from build123d import *

# Parameters (mm, degrees)
SKETCH3_R               = 15.55
SKETCH3_R_2             = 8.15
BOSS_EXTRUDE4_DEPTH     = 6.5
SKETCH2_R               = 15.55
SKETCH2_R_2             = 8.15
BOSS_EXTRUDE5_DEPTH     = 6.5
CUT_EXTRUDE1_DEPTH      = 35.8
SKETCH5_R               = 1.6
CUT_EXTRUDE2_DEPTH      = 43.014818814
BOSS_EXTRUDE6_DEPTH     = 6.5
SKETCH9_W               = 6.5
SKETCH9_H               = 21.954006421
BOSS_EXTRUDE7_DEPTH     = 4
BOSS_EXTRUDE8_DEPTH     = 6.5
FILLET1_R               = 2
FILLET5_R               = 2
CUT_EXTRUDE3_DEPTH      = 47.905543459
BOSS_EXTRUDE10_START    = -6.5
SKETCH13_W              = 19.5
SKETCH13_H              = 7.8
BOSS_EXTRUDE10_DEPTH    = 35.8
FILLET3_R               = 2
SKETCH14_W              = 19.5
SKETCH14_H              = 5
BOSS_EXTRUDE11_DEPTH    = 5
CUT_EXTRUDE4_DEPTH      = 62.410850086
SKETCH20_W              = 19.5
SKETCH20_H              = 5
BOSS_EXTRUDE13_DEPTH    = 4.5
SKETCH21_R              = 1.6
CUT_EXTRUDE7_DEPTH      = 62.410850086
FILLET6_R               = 1
SKETCH22_R              = 2.35
CUT_EXTRUDE8_DEPTH      = 10
SKETCH23_R              = 1.6
CUT_EXTRUDE9_DEPTH      = 54.54433838
CUT_EXTRUDE9_DEPTH_BACK = 54.54433838


with BuildPart() as part:
    # Sketch3 → Boss-Extrude4 (new body)
    with BuildSketch(Plane(origin=(0, 0, 0), x_dir=(0, 0, -1), z_dir=(1, 0, 0))):
        with Locations(Location((0, 0, 0), (0, 0, 180))):
            Circle(SKETCH3_R)
        with Locations(Location((0, 0, 0), (0, 0, 180))):
            Circle(SKETCH3_R_2, mode=Mode.SUBTRACT)
    extrude(amount=BOSS_EXTRUDE4_DEPTH)


with BuildPart() as body_2:
    # Sketch2 → Boss-Extrude5 (new body)
    with BuildSketch(Plane(origin=(35.8, 0, 0), x_dir=(0, 0, -1), z_dir=(1, 0, 0))):
        Circle(SKETCH2_R)
        Circle(SKETCH2_R_2, mode=Mode.SUBTRACT)
    extrude(amount=-BOSS_EXTRUDE5_DEPTH)


with BuildPart() as cut_extrude1_tool:
    # Sketch4 → Cut-Extrude1 (new body)
    with BuildSketch(Plane(origin=(0, 0, 0), x_dir=(0, 0, -1), z_dir=(1, 0, 0))):
        with BuildLine():
            Line((0, 15.55), (0, -15.55))
            ThreePointArc((0, -15.55), (15.55, 0), (0, 15.55))
        make_face()
    extrude(amount=CUT_EXTRUDE1_DEPTH)


with BuildPart() as part_1:
    add(part.part)

    # Cut-Extrude1: cut by cut_extrude1_tool
    add(cut_extrude1_tool.part, mode=Mode.SUBTRACT)


with BuildPart() as body_2_1:
    add(body_2.part)

    # Cut-Extrude1: cut by cut_extrude1_tool
    add(cut_extrude1_tool.part, mode=Mode.SUBTRACT)


with BuildPart() as cut_extrude2_tool:
    # Sketch5 → Cut-Extrude2 (new, through all)
    with BuildSketch(Plane(origin=(0, 0, 0), x_dir=(-1, 0, 0), z_dir=(0, 0, -1))):
        with Locations((-32.55, 11.85)):
            Circle(SKETCH5_R)
        with Locations((-3.25, 11.85)):
            Circle(SKETCH5_R)
    extrude(amount=-CUT_EXTRUDE2_DEPTH)


with BuildPart() as part_2:
    add(part_1.part)

    # Cut-Extrude2: cut by cut_extrude2_tool
    add(cut_extrude2_tool.part, mode=Mode.SUBTRACT)

    # Sketch11 → Boss-Extrude8 (add)
    with BuildSketch(Plane.ZY):
        with BuildLine():
            ThreePointArc((15.5, -1.245993579), (10.545788255, -11.427547859), (0, -15.55))
            Line((0, -15.55), (0, -23.2))
            Line((0, -23.2), (19.5, -23.2))
            Line((19.5, -23.2), (19.5, -1.245993579))
            Line((19.5, -1.245993579), (15.5, -1.245993579))
        make_face()
    extrude(amount=-BOSS_EXTRUDE8_DEPTH)

    # Fillet5
    fillet5_edges = [part_2.edges().sort_by_distance(p)[0] for p in [
        (3.25, -1.245993579, 15.5),
    ]]
    fillet(fillet5_edges, radius=FILLET5_R)


with BuildPart() as body_2_2:
    add(body_2_1.part)

    # Cut-Extrude2: cut by cut_extrude2_tool
    add(cut_extrude2_tool.part, mode=Mode.SUBTRACT)

    # Sketch8 → Boss-Extrude6 (add)
    with BuildSketch(Plane.ZY.offset(-29.3)):
        with BuildLine():
            ThreePointArc((15.5, -11.330931118), (8.691551143, -17.120074145), (0, -19.2))
            Line((0, -19.2), (0, -23.2))
            Line((0, -23.2), (15.5, -23.2))
            Line((15.5, -23.2), (15.5, -11.330931118))
        make_face()
        with BuildLine():
            ThreePointArc((15.5, -1.245993579), (10.545788255, -11.427547859), (0, -15.55))
            Line((0, -15.55), (0, -19.2))
            ThreePointArc((0, -19.2), (8.691551143, -17.120074145), (15.5, -11.330931118))
            Line((15.5, -11.330931118), (15.5, -1.245993579))
        make_face()
    extrude(amount=-BOSS_EXTRUDE6_DEPTH)

    # Sketch9 → Boss-Extrude7 (add)
    with BuildSketch(Plane(origin=(0, 0, 15.5), x_dir=(-1, 0, 0), z_dir=(0, 0, -1))):
        with Locations((-32.55, -12.22299679)):
            Rectangle(SKETCH9_W, SKETCH9_H)
    extrude(amount=-BOSS_EXTRUDE7_DEPTH)

    # Fillet1
    fillet1_edges = [body_2_2.edges().sort_by_distance(p)[0] for p in [
        (32.55, -1.245993579, 15.5),
    ]]
    fillet(fillet1_edges, radius=FILLET1_R)


with BuildPart() as cut_extrude3_tool:
    # Sketch10 → Cut-Extrude3 (new, through all)
    with BuildSketch(Plane.ZY.offset(-35.8)):
        with BuildLine():
            Line((19.5, -1.245993579), (19.5, -3.212198374))
            ThreePointArc((19.5, -3.212198374), (18.924111949, -1.82188163), (17.533795206, -1.245993579))
            Line((17.533795206, -1.245993579), (19.5, -1.245993579))
        make_face()
    extrude(amount=CUT_EXTRUDE3_DEPTH)


with BuildPart() as part_3:
    add(part_2.part)

    # Cut-Extrude3: cut by cut_extrude3_tool
    add(cut_extrude3_tool.part, mode=Mode.SUBTRACT)



with BuildPart() as body_2_3:
    add(body_2_2.part)

    # Cut-Extrude3: cut by cut_extrude3_tool
    add(cut_extrude3_tool.part, mode=Mode.SUBTRACT)


with BuildPart() as part_4:
    add(part_3.part)

    add(body_2_3.part)  # Boss-Extrude10 merges body 2
    # Sketch13 → Boss-Extrude10 (add)
    with BuildSketch(Plane.ZY.offset(-29.3).offset(BOSS_EXTRUDE10_START)):
        with Locations((9.75, -27.1)):
            Rectangle(SKETCH13_W, SKETCH13_H)
    extrude(amount=BOSS_EXTRUDE10_DEPTH)

    # Fillet3
    fillet3_edges = [part_4.edges().sort_by_distance(p)[0] for p in [
        (6.5, -23.2, 9.75),
        (29.3, -23.2, 9.75),
    ]]
    fillet(fillet3_edges, radius=FILLET3_R)

    # Sketch14 → Boss-Extrude11 (add)
    with BuildSketch(Plane.ZY.offset(-35.8)):
        with Locations((9.75, -28.5)):
            Rectangle(SKETCH14_W, SKETCH14_H)
    extrude(amount=-BOSS_EXTRUDE11_DEPTH)

    # Sketch15 → Cut-Extrude4 (cut, through all)
    with BuildSketch(Plane(origin=(0, -26, 0), x_dir=(1, 0, 0), z_dir=(0, 1, 0))):
        with BuildLine():
            ThreePointArc((39.9, -9.75), (39.43137085, -8.61862915), (38.3, -8.15))
            Line((38.3, -8.15), (38.3, -11.35))
            ThreePointArc((38.3, -11.35), (39.43137085, -10.88137085), (39.9, -9.75))
        make_face()
        with BuildLine():
            Line((38.3, -11.35), (38.3, -8.15))
            ThreePointArc((38.3, -8.15), (36.7, -9.75), (38.3, -11.35))
        make_face()
    extrude(amount=-CUT_EXTRUDE4_DEPTH, mode=Mode.SUBTRACT)

    # Sketch20 → Boss-Extrude13 (add)
    with BuildSketch(Plane.ZY):
        with Locations((9.75, -28.5)):
            Rectangle(SKETCH20_W, SKETCH20_H)
    extrude(amount=BOSS_EXTRUDE13_DEPTH)

    # Sketch21 → Cut-Extrude7 (cut, through all)
    with BuildSketch(Plane(origin=(0, -26, 0), x_dir=(1, 0, 0), z_dir=(0, 1, 0))):
        with Locations(Location((-2.25, -9.75, 0), (0, 0, 270))):
            Circle(SKETCH21_R)
    extrude(amount=-CUT_EXTRUDE7_DEPTH, mode=Mode.SUBTRACT)

    # Fillet6
    fillet6_edges = [part_4.edges().sort_by_distance(p)[0] for p in [
        (0, 11.229228387, 10.756715569),
        (0, -1.82188163, 18.924111949),
        (29.3, -12.206099187, 19.5),
        (17.9, -23.2, 19.5),
        (6.5, -12.206099187, 19.5),
        (28.714213562, -22.614213562, 19.5),
        (7.085786438, -22.614213562, 19.5),
        (40.8, -28.5, 19.5),
        (38.3, -26, 19.5),
        (-2.25, -26, 19.5),
        (-4.5, -28.5, 19.5),
        (35.8, 11.229228387, 10.756715569),
        (29.3, 11.229228387, 10.756715569),
        (29.3, -0.690267327, 16.150294811),
        (35.8, -0.690267327, 16.150294811),
        (35.8, -14.606099187, 19.5),
        (35.8, -1.82188163, 18.924111949),
        (29.3, -1.82188163, 18.924111949),
        (0, -14.606099187, 19.5),
        (18.15, -31, 19.5),
        (6.5, -0.690267327, 16.150294811),
        (6.5, -1.82188163, 18.924111949),
        (6.5, 11.229228387, 10.756715569),
        (0, -0.690267327, 16.150294811),
    ]]
    fillet(fillet6_edges, radius=FILLET6_R)

    # Sketch22 → Cut-Extrude8 (cut)
    with BuildSketch(Plane(origin=(0, 0, 0), x_dir=(-1, 0, 0), z_dir=(0, 0, -1))):
        with Locations((-8.5, -27.1)):
            Circle(SKETCH22_R)
        with Locations((-27.3, -27.1)):
            Circle(SKETCH22_R)
    extrude(amount=-CUT_EXTRUDE8_DEPTH, mode=Mode.SUBTRACT)

    # Sketch23 → Cut-Extrude9 (cut, two sides)
    with BuildSketch(Plane.XY.offset(15.535641906)) as cut_extrude9_sk:
        with Locations((3.25, 0)):
            Circle(SKETCH23_R)
        with Locations((32.55, 0)):
            Circle(SKETCH23_R)
    extrude(amount=CUT_EXTRUDE9_DEPTH, mode=Mode.SUBTRACT)
    extrude(cut_extrude9_sk.sketch, amount=-CUT_EXTRUDE9_DEPTH_BACK, mode=Mode.SUBTRACT)


solid = part_4.part
Could you check a few things on this model? Use its own coordinates, in mm. A direction names the side the tool comes from. Round coordinates to 2 decimals unless told otherwise and drop trailing zeros. Order: outer loops, then holes, each group sorted by start corner. A loop starts at its lowest first (then second) coordinate and runs counter-clockwise, first axis right, second up.
(1) Please list where these lines run through material, in increasing order: line 1 along X through (y, z) = (0, 14); line 2 along X through (y, z) = (-9.5, 17.5); line 3 along Y through (x, z) = (8.5, 6.75).
Response values:
line 1: x = 0 to 1.65, 4.85 to 6.5, 29.3 to 30.95, 34.15 to 35.8
line 2: x = 0 to 6.5, 29.3 to 35.8
line 3: y = -31 to -29.45, -24.75 to -23.2
(2) Imagine slicing it at C-C (x = 3.25). Write out the boundary of the cut face in (y, z), plus the area to 3 significant figures.
Response values:
outline: (-31, 0) - (-8.15, 0) arc R8.15 cw to (-1.6, 7.99) - (-1.6, 18.66) arc R1.97 ccw to (-3.21, 19.5) - (-30, 19.5) arc R1 ccw to (-31, 18.5) - close; (1.6, 7.99) arc R8.15 cw to (8.15, 0) - (10.25, 0) - (10.25, 11.69) arc R15.55 ccw to (1.6, 15.47) - close; (13.45, 0) - (15.55, 0) arc R15.55 ccw to (13.45, 7.8) - close
area: 627 mm2
(3) Imagine slicing it at D-D (z = 2.75). Count the separate pieces of the cut face and the enclosed holes in it, plus the area to 3 significant figures.
Response values:
separate pieces: 3
enclosed holes: 4
area: 578 mm2
(4) I'm going to push flat-ended pins straight in: pin 1 (9 mm diameter, centred on y = -10, z = 6.5, fed in from -X); pin 2 (8 mm diameter, centred on y = -11, z = 10, fed in from +X); pin 3 (1 mm diameter, centred on x = 36, y = -3, fed in from -Z); pin 4 (8 mm diameter, centred on x = 12, y = -14.5, fed in from -Z). Where does each tip first touch, or does it pass through?
Response values:
pin 1: stops at x = 0
pin 2: stops at x = 35.8
pin 3: stops at z = 7.38
pin 4: passes through
(5) Which directions (+Z, -Z, +X, -X, +Y, -Y) give clear straight access to the entire face, cutting with the end or side of a thin tool? Please do faces 1 (the flat face through (6.5, -7, 9)), 2 (the cylindrical face through (10.365, -28.53, 4.93)), 3 (the flat face through (0, -10, 9)).
Response values:
face 1: +Z, -Z, +Y
face 2: -Z
face 3: +Z, -Z, -X, +Y
(6) Imagine slicing it at A-A (x = -2.25). Write out the boundary of the cut face in (y, z).
Response values:
outline: (-31, 0) - (-26, 0) - (-26, 8.15) - (-31, 8.15) - close; (-31, 11.35) - (-26, 11.35) - (-26, 18.5) arc R1 ccw to (-27, 19.5) - (-30, 19.5) arc R1 ccw to (-31, 18.5) - close
(7) Imagine slicing it at B-B (y = -18). Write out the boundary of the cut face in (x, z), plus the area to 3 significant figures.
Response values:
outline: (0, 0) - (6.5, 0) - (6.5, 18.5) arc R1 ccw to (5.5, 19.5) - (1, 19.5) arc R1 ccw to (0, 18.5) - close; (29.3, 0) - (35.8, 0) - (35.8, 18.5) arc R1 ccw to (34.8, 19.5) - (30.3, 19.5) arc R1 ccw to (29.3, 18.5) - close
area: 253 mm2
(8) If we mould it in two halves opening along X, with no side actions, what happens to faces 4 (the cylindrical face through (25.13, -28, 4.93)), 5 (the flat face through (18, -31, 9)), 6 (the flat face through (40.8, -28, 9))? For each: released by +X, released by -X, zero draft, split by the parting line, or undercut.
Response values:
face 4: undercut
face 5: zero draft
face 6: released by +X
